Source: CAD feature listing. Evaluate the final solid. Frame: model axes, mm. Give positions to 0.01 mm unless a question says otherwise; leave off trailing zeros. Write each loop counter-clockwise with the first axis right and the second up, starting at its lowest first coordinate (ties: lowest second). Pieces come first, ordered by that corner, then holes. Notation, with made-up numbers: (6, 86) -> (43, 86) arc R14 ccw to (43, 103) -> close; hole circle Ø3 at (31.5, 27.25). An arc over 180 degrees is marked (long way). Use one line per item in the form item = value. Start each with the question number.
(1) Cut plane C-C, the plane z = 0.8. Output: boundary loops of the cut face in (x, y), and give its area (3 significant figures).
(2) Material intervals for line 1 along X through (y, z) = (-18.5, 0.7); line 2 along X through (y, z) = (19.5, 0.7); line 3 along X through (y, z) = (4.5, 0.3), sorted ascending. Write a range as from..to.
(3) Cut plane A-A, the plane x = -19.5. Output: boundary loops of the cut face in (y, z), and give its area (3 significant figures).
(4) First-contact query: P1, Ø2, axis at x = 1.5, y = 11, coming from the -Z side. Flat tip, straight axial feed; report the tip coordinate or a pass-through.
from build123d import *

# Parameters (mm, degrees)
ESQUISSE3_W                                 = 44
ESQUISSE3_H                                 = 44
BOSS_EXTRU_1_DEPTH                          = 1
SKETCH_HOLES_R                              = 0.5
CUT_EXTRUDE_HOLES_DEPTH                     = 2
FRAISAGE_POUR_VIS_T_TE_FRAIS_E_M21_AT_COUNT = 2
FRAISAGE_POUR_VIS_T_TE_FRAIS_E_M21_AT_PITCH = 39
FRAISAGE_POUR_VIS_T_TE_FRAIS_E_M21_2_COUNT  = 2
FRAISAGE_POUR_VIS_T_TE_FRAIS_E_M21_2_PITCH  = 55.154328933
FRAISAGE_POUR_VIS_T_TE_FRAIS_E_M21_3_COUNT  = 2
FRAISAGE_POUR_VIS_T_TE_FRAIS_E_M21_3_PITCH  = 39


with BuildPart() as part:
    # Esquisse3 → Boss.-Extru.1 (new body)
    with BuildSketch(Plane(origin=(0, 0, 0), x_dir=(0, 1, 0), z_dir=(0, 0, 1))):
        Rectangle(ESQUISSE3_W, ESQUISSE3_H)
    extrude(amount=BOSS_EXTRU_1_DEPTH)

    # Sketch_Holes → Cut_Extrude_Holes (cut, through all)
    with BuildSketch(Plane.XY.offset(1)):
        with Locations((-10.067654011, 4.160184375)):
            Circle(SKETCH_HOLES_R)
    extrude(amount=-CUT_EXTRUDE_HOLES_DEPTH, mode=Mode.SUBTRACT)

    # Esquisse5 → Fraisage pour vis à tête fraisée M21 (revolve, cut)
    with BuildSketch(Plane(origin=(19.5, -19.5, 1), x_dir=(0, -1, 0), z_dir=(1, 0, 0))):
        Polygon((0, 0), (0, 2), (1.2, 2), (1.2, 1), (2.2, 0), align=None)
    fraisage_pour_vis_t_te_frais_e_m21 = revolve(axis=Axis((19.5, -19.5, 7.35), (0, 0, -1)), mode=Mode.SUBTRACT)

    # Fraisage pour vis à tête fraisée M21 at: Fraisage pour vis à tête fraisée M21 ×2
    with Locations(*[(-i * FRAISAGE_POUR_VIS_T_TE_FRAIS_E_M21_AT_PITCH, 0, 0) for i in range(1, FRAISAGE_POUR_VIS_T_TE_FRAIS_E_M21_AT_COUNT)]):
        add(fraisage_pour_vis_t_te_frais_e_m21, mode=Mode.SUBTRACT)

    # Fraisage pour vis _ t_te frais_e M21 2: Fraisage pour vis à tête fraisée M21 ×2
    with Locations(*[Vector(-0.707106781, 0.707106781, 0) * (i * FRAISAGE_POUR_VIS_T_TE_FRAIS_E_M21_2_PITCH) for i in range(1, FRAISAGE_POUR_VIS_T_TE_FRAIS_E_M21_2_COUNT)]):
        add(fraisage_pour_vis_t_te_frais_e_m21, mode=Mode.SUBTRACT)

    # Fraisage pour vis _ t_te frais_e M21 3: Fraisage pour vis à tête fraisée M21 ×2
    with Locations(*[(0, i * FRAISAGE_POUR_VIS_T_TE_FRAIS_E_M21_3_PITCH, 0) for i in range(1, FRAISAGE_POUR_VIS_T_TE_FRAIS_E_M21_3_COUNT)]):
        add(fraisage_pour_vis_t_te_frais_e_m21, mode=Mode.SUBTRACT)


solid = part.part
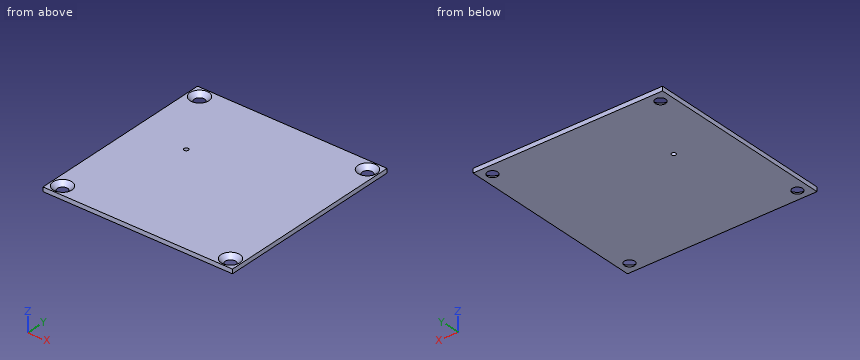
Geometry says:
q1.outline = (-22, -22) -> (22, -22) -> (22, 22) -> (-22, 22) -> close; hole circle Ø4 at (-19.5, -19.5); hole circle Ø4 at (-19.5, 19.5); hole circle Ø1 at (-10.07, 4.16); hole circle Ø4 at (19.5, -19.5); hole circle Ø4 at (19.5, 19.5)
q1.area = 1,880 mm^2
q2.line_1 = -22..-21.12, -17.88..17.88, 21.12..22
q2.line_2 = -22..-21.4, -17.6..17.6, 21.4..22
q2.line_3 = -22..-10.43, -9.7..22
q3.outline = (-22, 0) -> (-20.7, 0) -> (-21.7, 1) -> (-22, 1) -> close; (-18.3, 0) -> (18.3, 0) -> (17.3, 1) -> (-17.3, 1) -> close; (20.7, 0) -> (22, 0) -> (22, 1) -> (21.7, 1) -> close
q3.area = 37.2 mm^2
q4.P1 = 0
